CAD build for the part. Positions are in the model's coordinates, mm. Give positions to 0.01 mm unless a question says otherwise; leave off trailing zeros. Write each loop counter-clockwise with the first axis right and the second up, starting at its lowest first coordinate (ties: lowest second). Pieces come first, ordered by that corner, then holes. Notation, with made-up numbers: (52.5, 5.5) -> (57.5, 5.5) arc R24 ccw to (57.5, 18.5) -> close; hole circle Ø5 at (49.5, 13.25). An arc over 180 degrees is marked (long way). Answer as a JSON object with one key per item and string values.
Autodesk Inventor part; units mm, degrees
ref_plane "YZ Plane" through (0, 0, 0) normal (1, 0, 0) x (0, 1, 0)
ref_plane "XZ Plane" through (0, 0, 0) normal (0, 1, 0) x (-1, 0, 0)
ref_plane "XY Plane" through (0, 0, 0) normal (0, 0, 1) x (1, 0, 0)
sketch "Esboço1" plane through (0, 0, 0) normal (0, 1, 0) x (-1, 0, 0)
  circle A0 centre (0, 0) radius 32.5
  circle A1 centre (0, 0) radius 1.5
  dimension "d0" = 65
  dimension "d3" = 3
extrude "Extrusão1" add sketch "Esboço1" along normal blind 12
sketch "Esboço2" plane through (0, 0, 0) normal (0, -1, 0) x (1, 0, 0)
  circle A0 centre (0, 0) radius 1.5
  circle A1 centre (0, 0) radius 26
  circle A2 centre (0, -26) radius 2.1
  circle A3 centre (0, 26) radius 2.1
  dimension "d4" = 4.2
  dimension "d5" = 4.2
  dimension "d11" = 52
extrude "Extrusão2" cut sketch "Esboço2" against normal blind 12 contours A3 A1 | A1 A3 | A2 A1 | A1 A2
chamfer "Chanfro1" distance 2.5 angle 45 2 edges at (-2.1, 0, 26) (-2.1, 0, -26)
properties part number "Inferior_encaixe"
1) Slice it at D-D (z = -12.5). List the corners of the cut face in (x, y), then the cut area to 3 significant figures.
Model answer:
{"outline": "(-30, 0) -> (30, 0) -> (30, 12) -> (-30, 12) -> close", "area": "720 mm2"}
2) Slice it at A-A (z = 26). List the corners of the cut face in (x, y), then the cut area to 3 significant figures.
Model answer:
{"outline": "(-19.5, 0) -> (-4.6, 0) -> (-2.1, 2.5) -> (-2.1, 12) -> (-19.5, 12) -> close; (2.1, 2.5) -> (4.6, 0) -> (19.5, 0) -> (19.5, 12) -> (2.1, 12) -> close", "area": "411 mm2"}
3) Slice it at C-C (y = 7.25). List the corners of the cut face in (x, z), then the cut area to 3 significant figures.
Model answer:
{"outline": "circle Ø65 at (0, 0); hole circle Ø4.2 at (0, -26); hole circle Ø4.2 at (0, 26); hole circle Ø3 at (0, 0)", "area": "3,280 mm2"}
4) Mould opens along X. For faces 1 (the conical face through (-0.489, 2.344, 23.797)), 2 (the cylindrical face through (-31, 5.92, -9.76)), 3 (the cylindrical face through (1.13, 7.18, -24.23)), 4 (the flat face through (-7, 12, 0)) say: released by +X, released by -X, zero draft, split by the parting line, or undercut.
Model answer:
{"face 1": "undercut", "face 2": "split by the parting line", "face 3": "undercut", "face 4": "zero draft"}
5) Wall check: probe 1 along Z at (x, y) = (0, 6); probe 2 along X at (y, z) = (11, 27); probe 3 along X at (y, z) = (5, -26). Give the ranges that are in metal, low to high.
Model answer:
{"probe 1": "z = -32.5 to -28.1, -23.9 to -1.5, 1.5 to 23.9, 28.1 to 32.5", "probe 2": "x = -18.09 to -1.85, 1.85 to 18.09", "probe 3": "x = -19.5 to -2.1, 2.1 to 19.5"}
6) Pin check, flat tips, straight feed: pin 1 (3 mm diameter, centred on x = 13, y = 2, fed in from -Z); pin 2 (5 mm diameter, centred on y = 9, z = 21.5, fed in from -X); pin 3 (1 mm diameter, centred on y = 7.5, z = -12.5, fed in from +X); pin 4 (3.5 mm diameter, centred on x = 0, z = 26, fed in from +Y). Stop position of each tip, or through.
Model answer:
{"pin 1": "stops at z = -30.4", "pin 2": "stops at x = -26.37", "pin 3": "stops at x = 30.2", "pin 4": "passes through"}
7) Slice it at B-B (x = 0). List the corners of the cut face in (y, z), then the cut area to 3 significant figures.
Model answer:
{"outline": "(0, -32.5) -> (12, -32.5) -> (12, -28.1) -> (2.5, -28.1) -> (0, -30.6) -> close; (0, -21.4) -> (2.5, -23.9) -> (12, -23.9) -> (12, -1.5) -> (0, -1.5) -> close; (0, 1.5) -> (12, 1.5) -> (12, 23.9) -> (2.5, 23.9) -> (0, 21.4) -> close; (0, 30.6) -> (2.5, 28.1) -> (12, 28.1) -> (12, 32.5) -> (0, 32.5) -> close", "area": "631 mm2"}
